The listing builds one solid part. Answer for the finished solid, in the listing's coordinates (mm). A direction names the side the tool comes from. Coordinates: 2 decimals unless noted, no trailing zeros. Loops run counter-clockwise (first coordinate to the right, second up) from the corner with the lowest first, then second, coordinate; pieces in that order, holes last. Notation, with made-up numbers: (-24, 28) - (33, 28) arc R17 ccw to (33, 37) - close; hole circle Ø10 at (62, 1). An arc over 180 degrees is marked (long way). Return JSON: item names as keys, results as strings. Group by question number.
1. Section D-D (y = -6.5) is taken. Write down the section's boundary in (x, z).
2. The mould has two halves that part along Y. Classify faces 1 (the face through (-1.7, 3.8, 2.5)), 2 (the face through (-2.17, 9.76, 1.48)), 3 (the face through (4.3, -2.1, 3)): pulls with the +Y half, pulls with the -Y half, needs draft (parallel to the pull), parting line crosses it, or undercut.
3. Section C-C (x = 7) is taken. Write down the section's boundary in (y, z), and give its area (3 significant figures).
4. Each of these flat-tipped pins is pushed along its axis until it touches: P1, Ø2.5, axis at x = 4.95, y = 4.95, coming from the -Z side; P2, Ø1, axis at x = 5, z = 1.5, coming from the -Y side; P3, Ø1, axis at y = -6.5, z = 2.5, coming from the +X side. Where does it stop, or does it pass through?
5. Find the intervals of material crossed by line 1 along Y through (x, z) = (1.75, 2.65); line 2 along X through (y, z) = (-6.5, 1.1); line 3 along Z through (x, y) = (0, -4.25), in increasing order.
6. Section A-A (y = 0) is taken. Write down the section's boundary in (x, z), and give its area (3 significant figures).
7. Which of the six approach directions +Z, -Z, +X, -X, +Y, -Y give full straight-line access (tool end or side, diameter ignored) to faces 4 (the face through (4.3, 0.1, 0)), 5 (the face through (-3.65, -2.8, 2.75))?
Autodesk Inventor part; units mm, degrees
ref_plane "YZ Plane" through (0, 0, 0) normal (1, 0, 0) x (0, 1, 0)
ref_plane "XZ Plane" through (0, 0, 0) normal (0, 1, 0) x (-1, 0, 0)
ref_plane "XY Plane" through (0, 0, 0) normal (0, 0, 1) x (1, 0, 0)
sketch "スケッチ1" plane through (0, 0, 0) normal (0, 0, 1) x (1, 0, 0)
  circle A0 centre (0, 0) radius 10
  dimension "d0" = 20
extrude "押し出し1" add sketch "スケッチ1" along normal blind 3
sketch "スケッチ5" plane through (0, 0, 3) normal (0, 0, 1) x (1, 0, 0)
  circle A0 centre (0, 7) radius 1
  circle A1 centre (0, 0) radius 10
  dimension "d30" = 2
  dimension "d77" = 0
  dimension "d78" = 7
hole "穴4" at (0, 7, 3) direction (0, 0, -1) diameter 1.941 end through all
sketch "スケッチ6" plane through (0, 0, 0) normal (0, 0, -1) x (-1, 0, 0)
  circle A0 centre (0, 0) radius 10
  circle A1 centre (0, 0) radius 4.05
  dimension "d66" = 8.1
hole "穴5" at (0, 0, 0) direction (0, 0, 1) diameter 8 end through all
sketch "スケッチ2" plane through (0, 0, 3) normal (0, 0, 1) x (1, 0, 0)
  circle A0 centre (0, 0) radius 10
  circle A1 centre (0, 0) radius 4.6
  dimension "d3" = 9.2
extrude "押し出し4" cut sketch "スケッチ2" against normal blind 0.5 contours A1
pattern_circular "円形状パターン3" count 8 over 360 about axis through (0, 0, 28.4429) along (0, 0, -1) of "穴4"
properties part number "03" material "アルミニウム 6061"
The answers:
{
 "1": {"outline": "(-7.6, 0) - (-0.83, 0) - (-0.83, 3) - (-7.6, 3) - close; (0.83, 0) - (7.6, 0) - (7.6, 3) - (0.83, 3) - close"},
 "2": {"face 1": "undercut", "face 2": "parting line crosses it", "face 3": "needs draft"},
 "3": {"outline": "(-7.14, 0) - (-0.97, 0) - (-0.97, 3) - (-7.14, 3) - close; (0.97, 0) - (7.14, 0) - (7.14, 3) - (0.97, 3) - close", "area": "37.0 mm2"},
 "4": {"P1": "stops at z = 0", "P2": "stops at y = -8.93", "P3": "stops at x = 8"},
 "5": {"line 1": "y = -9.85 to -4.25, 4.25 to 9.85", "line 2": "x = -7.6 to -0.83, 0.83 to 7.6", "line 3": "z = 0 to 2.5"},
 "6": {"outline": "(-10, 0) - (-7.97, 0) - (-7.97, 3) - (-10, 3) - close; (-6.03, 0) - (-4, 0) - (-4, 2.5) - (-4.6, 2.5) - (-4.6, 3) - (-6.03, 3) - close; (4, 0) - (6.03, 0) - (6.03, 3) - (4.6, 3) - (4.6, 2.5) - (4, 2.5) - close; (7.97, 0) - (10, 0) - (10, 3) - (7.97, 3) - close", "area": "23.8 mm2"},
 "7": {"face 4": "-Z, +X, -X, +Y, -Y", "face 5": "+Z"}
}
